from build123d import *

# Parameters (mm, degrees)
MODEL_W                 = 3
MODEL_H                 = 3
SALIENTE_EXTRUIR1_DEPTH = 3


with BuildPart() as part:
    # Model → Saliente-Extruir1 (new body)
    with BuildSketch(Plane.XY):
        with BuildLine():
            Line((9.925690899, 288.164372243), (8.925690899, 289.164372243))
            Line((8.925690899, 289.164372243), (9.925690899, 290.164372243))
            Line((9.925690899, 290.164372243), (14.425690899, 290.164372243))
            ThreePointArc((14.425690899, 290.164372243), (17.607671414, 288.846352758), (18.925690899, 285.664372243))
            Line((18.925690899, 285.664372243), (18.925690899, 258.664372243))
            ThreePointArc((18.925690899, 258.664372243), (17.607671414, 255.482391728), (14.425690899, 254.164372243))
            Line((14.425690899, 254.164372243), (9.925690899, 254.164372243))
            Line((9.925690899, 254.164372243), (8.925690899, 255.164372243))
            Line((8.925690899, 255.164372243), (9.925690899, 256.164372243))
            Line((9.925690899, 256.164372243), (8.925690899, 257.164372243))
            Line((8.925690899, 257.164372243), (9.925690899, 258.164372243))
            Line((9.925690899, 258.164372243), (8.925690899, 259.164372243))
            Line((8.925690899, 259.164372243), (9.925690899, 260.164372243))
            Line((9.925690899, 260.164372243), (8.925690899, 261.164372243))
            Line((8.925690899, 261.164372243), (9.925690899, 262.164372243))
            Line((9.925690899, 262.164372243), (8.925690899, 263.164372243))
            Line((8.925690899, 263.164372243), (9.925690899, 264.164372243))
            Line((9.925690899, 264.164372243), (8.925690899, 265.164372243))
            Line((8.925690899, 265.164372243), (9.925690899, 266.164372243))
            Line((9.925690899, 266.164372243), (8.925690899, 267.164372243))
            Line((8.925690899, 267.164372243), (9.925690899, 268.164372243))
            Line((9.925690899, 268.164372243), (8.925690899, 269.164372243))
            Line((8.925690899, 269.164372243), (9.925690899, 270.164372243))
            Line((9.925690899, 270.164372243), (8.925690899, 271.164372243))
            Line((8.925690899, 271.164372243), (9.925690899, 272.164372243))
            Line((9.925690899, 272.164372243), (8.925690899, 273.164372243))
            Line((8.925690899, 273.164372243), (9.925690899, 274.164372243))
            Line((9.925690899, 274.164372243), (8.925690899, 275.164372243))
            Line((8.925690899, 275.164372243), (9.925690899, 276.164372243))
            Line((9.925690899, 276.164372243), (8.925690899, 277.164372243))
            Line((8.925690899, 277.164372243), (9.925690899, 278.164372243))
            Line((9.925690899, 278.164372243), (8.925690899, 279.164372243))
            Line((8.925690899, 279.164372243), (9.925690899, 280.164372243))
            Line((9.925690899, 280.164372243), (8.925690899, 281.164372243))
            Line((8.925690899, 281.164372243), (9.925690899, 282.164372243))
            Line((9.925690899, 282.164372243), (8.925690899, 283.164372243))
            Line((8.925690899, 283.164372243), (9.925690899, 284.164372243))
            Line((9.925690899, 284.164372243), (8.925690899, 285.164372243))
            Line((8.925690899, 285.164372243), (9.925690899, 286.164372243))
            Line((9.925690899, 286.164372243), (8.925690899, 287.164372243))
            Line((8.925690899, 287.164372243), (9.925690899, 288.164372243))
        make_face()
        with Locations((14.425690899, 285.664372243)):
            Rectangle(MODEL_W, MODEL_H, mode=Mode.SUBTRACT)
        with Locations((14.425690899, 276.664372243)):
            Rectangle(MODEL_W, MODEL_H, mode=Mode.SUBTRACT)
        with Locations((14.425690899, 258.664372243)):
            Rectangle(MODEL_W, MODEL_H, mode=Mode.SUBTRACT)
        with Locations((14.425690899, 267.664372243)):
            Rectangle(MODEL_W, MODEL_H, mode=Mode.SUBTRACT)
    extrude(amount=SALIENTE_EXTRUIR1_DEPTH)


solid = part.part
Verification items for the finished model (mm, model axes). A direction names the side the tool comes from. Round coordinates to 2 decimals unless told otherwise and drop trailing zeros. Loops run counter-clockwise (first coordinate to the right, second up) from the corner with the lowest first, then second, coordinate; pieces in that order, holes last. Notation, with made-up numbers: (37, -20) - (89, -20) arc R22 cw to (89, -3) - close; hole circle Ø10 at (-14, 68). An arc over 180 degrees is marked (long way). Answer in a Markdown table with one row per item. Add a question column.
Q1. Material ranges on line 1 (Y direction, x = 14, z = 1.9); line 2 (Y direction, x = 15.75, z = 2.85); line 3 (X direction, y = 278, z = 0.7), recorded low to high.
Q2. Tool access check on faces 5 (the face through (12, 290.164, 1)), 6 (the face through (9.42, 261.66, 1.48)), 7 (the face through (15.926, 268, 1)). Record the directions out of +Z, -Z, +X, -X, +Y, -Y that give a thin tool (end or side, any length) a straight path to the whole face; none if there is none.
Q3. Section check A-A on y = 276.5. Enter the section's corners in (x, z), plus the area to 3 significant figures.
Q4. Section check C-C on x = 18. Enter the section's corners in (y, z).
Q5. Section check B-B on z = 0.7. State how many separate pieces and enclosed holes the cut face has, plus the area to 3 significant figures.
Q6. Release check for a two-part mould opening along Y. For faces 1 (the face through (12, 254.164, 1)), 2 (the face through (9.42, 255.66, 1.48)), 3 (the face through (9.42, 257.66, 1.48)), 4 (the face through (14, 272, 3)) record: pulls with the +Y half, pulls with the -Y half, needs draft (parallel to the pull), parting line crosses it, or undercut.
Found:
| question | item | result |
|---|---|---|
| 1 | line 1 | y = 254.16 to 257.16, 260.16 to 266.16, 269.16 to 275.16, 278.16 to 284.16, 287.16 to 290.16 |
| 1 | line 2 | y = 254.36 to 257.16, 260.16 to 266.16, 269.16 to 275.16, 278.16 to 284.16, 287.16 to 289.97 |
| 1 | line 3 | x = 9.76 to 12.93, 15.93 to 18.93 |
| 2 | face 5 | +Z, -Z, +X, -X, +Y |
| 2 | face 6 | +Z, -Z, -X |
| 2 | face 7 | +Z, -Z |
| 3 | outline | (9.59, 0) - (12.93, 0) - (12.93, 3) - (9.59, 3) - close; (15.93, 0) - (18.93, 0) - (18.93, 3) - (15.93, 3) - close |
| 3 | area | 19.0 mm² |
| 4 | outline | (255.93, 0) - (288.4, 0) - (288.4, 3) - (255.93, 3) - close |
| 5 | separate pieces | 1 |
| 5 | enclosed holes | 4 |
| 5 | area | 297 mm² |
| 6 | face 1 | pulls with the -Y half |
| 6 | face 2 | undercut |
| 6 | face 3 | undercut |
| 6 | face 4 | needs draft |
